```python
from build123d import *

# Parameters (mm, degrees)
F0_R     = 63.5
F1_DEPTH = 76.2
F3_R     = 48.310271
F4_DEPTH = 2.286
F5_W     = 67.779378
F5_H     = 33.0435
F6_DEPTH = 127


with BuildPart() as f1:
    # F0 (on Top) → F1 (new body)
    with BuildSketch(Plane.XY):
        Circle(F0_R)
    extrude(amount=F1_DEPTH)

    # F3 (on face) → F4 (join)
    with BuildSketch(Plane.XY.offset(76.2)):
        Circle(F3_R)
    extrude(amount=F4_DEPTH)

    # F5 (on Front) → F6 (cut)
    with BuildSketch(Plane.XZ):
        with Locations((0, 37.875455)):
            Rectangle(F5_W, F5_H)
    extrude(amount=F6_DEPTH, mode=Mode.SUBTRACT)


solid = f1.part
```
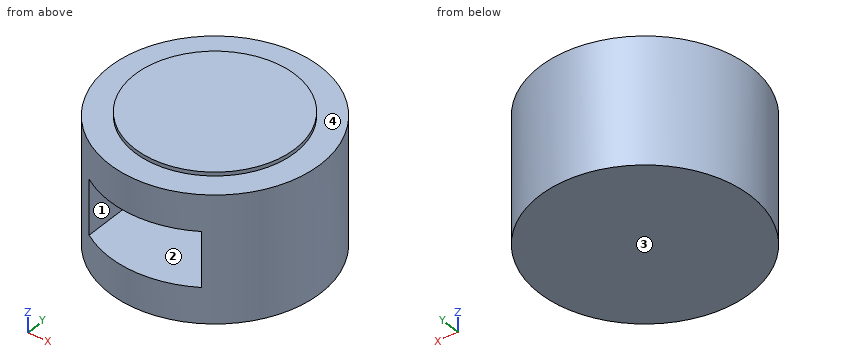
The listing builds one solid part. Answer for the finished solid, in the listing's coordinates (mm). Face numbers are marked on the shaded views. Round coordinates to 2 decimals unless told otherwise and drop trailing zeros. Order: outer loops, then holes, each group sorted by start corner. A loop starts at its lowest first (then second) coordinate and runs counter-clockwise, first axis right, second up. Notation, with made-up numbers: (-4, 68) -> (52, 68) arc R23 cw to (52, 97) -> close; hole circle Ø3 at (2, 35.25). An arc over 180 degrees is marked (long way). Answer as CSV lines item,"result". Start each with the question number.
(1) Flat-ended cylindrical pins translate along their axes: pin 1 Ø2 at (y, z) = (39.5, 37) entering from +X; pin 2 Ø1.5 at (x, y) = (-12.5, -47.5) entering from +Z; pin 3 Ø8 at (y, z) = (48, 16.5) entering from -X. Find the tip coordinate at first contact, or state that the pin passes through.
(2) For a pull along Z with two mould halves and no side action, classify the marked faces 1, 2, 3 and 4 as +Z half, -Z half, draft (parallel to the pull), parting line (faces both ways), or undercut.
(3) The part is cut by section B-B (y = -38.5). Determine the outline of the cut face in (x, z).
(4) The part is cut by section A-A (x = 0). Determine the outline of the cut face in (y, z).
(5) The part is cut by section C-C (z = 44.5). Determine the outline of the cut face in (x, y).
(6) The part is cut by section D-D (y = 34.5). Determine the outline of the cut face in (x, z), then the cut area to 3 significant figures.
(7) Find the intervals of material crossed by probe 1 along Z at (x, y) = (2, -53.5); probe 2 along Z at (x, y) = (-43.5, -35); probe 3 along X at (y, z) = (-2.5, 49.5), in increasing order. Write a range as from..to.
Evaluation:
1,pin 1,"x = 50.5"
1,pin 2,"z = 76.2"
1,pin 3,"x = -45.78"
2,face 1,"undercut"
2,face 2,"undercut"
2,face 3,"-Z half"
2,face 4,"+Z half"
3,outline,"(-50.5, 0) -> (50.5, 0) -> (50.5, 76.2) -> (29.18, 76.2) -> (29.18, 78.49) -> (-29.18, 78.49) -> (-29.18, 76.2) -> (-50.5, 76.2) -> close; hole (-33.89, 21.35) -> (33.89, 21.35) -> (33.89, 54.4) -> (-33.89, 54.4) -> close"
4,outline,"(-63.5, 0) -> (63.5, 0) -> (63.5, 76.2) -> (48.31, 76.2) -> (48.31, 78.49) -> (-48.31, 78.49) -> (-48.31, 76.2) -> (-63.5, 76.2) -> (-63.5, 54.4) -> (0, 54.4) -> (0, 21.35) -> (-63.5, 21.35) -> close"
5,outline,"(-33.89, -53.7) -> (-33.89, 0) -> (33.89, 0) -> (33.89, -53.7) arc R63.5 ccw (long way) to start"
6,outline,"(-53.31, 0) -> (53.31, 0) -> (53.31, 76.2) -> (33.82, 76.2) -> (33.82, 78.49) -> (-33.82, 78.49) -> (-33.82, 76.2) -> (-53.31, 76.2) -> close"
6,area,"8,280 mm²"
7,probe 1,"0..21.35, 54.4..76.2"
7,probe 2,"0..76.2"
7,probe 3,"-63.45..-33.89, 33.89..63.45"
